from build123d import *

# Parameters (mm, degrees)
F1_DEPTH  = 20
F2_START  = 10
F1_FACE_R = 1.5
F2_DEPTH  = 10


# Not quite as in the source:
# - a feature names something its author has since deleted; it is built from what else it names


with BuildPart() as f1:
    # F0 (on Top) → F1 (new body)
    with BuildSketch(Plane.XY):
        Polygon((8, 0), (0, 0), (0, -2), (10, -2), (10, 4), (10, 10), (0, 10), (0, 8), (8, 8), align=None)
        with BuildLine():
            Line((16, 2.5), (16, -2))
            ThreePointArc((16, -2), (22, 4), (16, 10))
            Line((16, 10), (16, 5.5))
            ThreePointArc((16, 5.5), (17.0606601718, 5.0606601718), (17.5, 4))
            ThreePointArc((17.5, 4), (17.0606601718, 2.9393398282), (16, 2.5))
        make_face()
        with BuildLine():
            ThreePointArc((10, 4), (11.7573593129, -0.2426406871), (16, -2))
            Line((16, -2), (16, 2.5))
            ThreePointArc((16, 2.5), (14.5, 4), (16, 5.5))
            Line((16, 5.5), (16, 10))
            ThreePointArc((16, 10), (11.7573593129, 8.2426406871), (10, 4))
        make_face()
        with BuildLine():
            Line((16, 10), (10, 10))
            Line((10, 10), (10, 4))
            ThreePointArc((10, 4), (11.7573593129, 8.2426406871), (16, 10))
        make_face()
        with BuildLine():
            Line((10, 4), (10, -2))
            Line((10, -2), (16, -2))
            ThreePointArc((16, -2), (11.7573593129, -0.2426406871), (10, 4))
        make_face()
    extrude(amount=F1_DEPTH)

    # F0 (on Top) + F1_face (on face) → F2 (cut)
    with BuildSketch(Plane.XY.offset(F2_START)):
        with BuildLine():
            Line((16, 2.5), (16, -2))
            ThreePointArc((16, -2), (22, 4), (16, 10))
            Line((16, 10), (16, 5.5))
            ThreePointArc((16, 5.5), (17.0606601718, 5.0606601718), (17.5, 4))
            ThreePointArc((17.5, 4), (17.0606601718, 2.9393398282), (16, 2.5))
        make_face()
        with BuildLine():
            ThreePointArc((10, 4), (11.7573593129, -0.2426406871), (16, -2))
            Line((16, -2), (16, 2.5))
            ThreePointArc((16, 2.5), (14.5, 4), (16, 5.5))
            Line((16, 5.5), (16, 10))
            ThreePointArc((16, 10), (11.7573593129, 8.2426406871), (10, 4))
        make_face()
        with BuildLine():
            Line((10, 4), (10, -2))
            Line((10, -2), (16, -2))
            ThreePointArc((16, -2), (11.7573593129, -0.2426406871), (10, 4))
        make_face()
        with BuildLine():
            Line((16, 10), (10, 10))
            Line((10, 10), (10, 4))
            ThreePointArc((10, 4), (11.7573593129, 8.2426406871), (16, 10))
        make_face()
    with BuildSketch(Plane(origin=(12.4841125556, 4, 20), x_dir=(1, 0, 0), z_dir=(0, 0, 1)).offset(F2_START)):
        with BuildLine():
            Line((-4.4841125556, -4), (-12.4841125556, -4))
            Line((-12.4841125556, -4), (-12.4841125556, -6))
            Line((-12.4841125556, -6), (3.5158874444, -6))
            ThreePointArc((3.5158874444, -6), (9.5158874444, 0), (3.5158874444, 6))
            Line((3.5158874444, 6), (-12.4841125556, 6))
            Line((-12.4841125556, 6), (-12.4841125556, 4))
            Line((-12.4841125556, 4), (-4.4841125556, 4))
            Line((-4.4841125556, 4), (-4.4841125556, -4))
        make_face()
        with Locations((3.5158874444, 0)):
            Circle(F1_FACE_R, mode=Mode.SUBTRACT)
    extrude(amount=F2_DEPTH, mode=Mode.SUBTRACT)


solid = f1.part
Source: CAD feature listing. Evaluate the final solid. Frame: model axes, mm. A direction names the side the tool comes from. Give positions to 0.01 mm unless a question says otherwise; leave off trailing zeros. Order: outer loops, then holes, each group sorted by start corner. A loop starts at its lowest first (then second) coordinate and runs counter-clockwise, first axis right, second up. Notation, with made-up numbers: (58, 21) -> (78, 21) arc R18 ccw to (78, 39) -> close; hole circle Ø10 at (41, 35.5). An arc over 180 degrees is marked (long way). Write item = value, one per line.
Q1. Cut plane B-B, the plane x = 17. Output: boundary loops of the cut face in (y, z), and give its area (3 significant figures).
Data:
outline = (-1.92, 0) -> (2.88, 0) -> (2.88, 10) -> (-1.92, 10) -> close; (5.12, 0) -> (9.92, 0) -> (9.92, 10) -> (5.12, 10) -> close
area = 96.0 mm^2
Q2. Set-up query: faces 1 (the face through (8, 4, 10)), 2 (the face through (10, 4, 15)), 3 (the face through (8.3, 5.4, 20)). Return all of +Z, -Z, +X, -X, +Y, -Y with unobstructed straight access to the full face (end or side cutting, diameter ignored); none if empty.
Data:
face_1 = +Z, -Z, -X
face_2 = +Z, +X, +Y, -Y
face_3 = +Z, +X, -X, +Y, -Y
Q3. Cut plane C-C, the plane z = 11. Output: boundary loops of the cut face in (x, y), and give its area (3 significant figures).
Data:
outline = (0, -2) -> (10, -2) -> (10, 10) -> (0, 10) -> (0, 8) -> (8, 8) -> (8, 0) -> (0, 0) -> close
area = 56.0 mm^2
Q4. Cut plane A-A, the plane z = 8.5. Output: boundary loops of the cut face in (x, y), and give its area (3 significant figures).
Data:
outline = (0, -2) -> (16, -2) arc R6 ccw to (16, 10) -> (0, 10) -> (0, 8) -> (8, 8) -> (8, 0) -> (0, 0) -> close; hole circle Ø3 at (16, 4)
area = 177 mm^2
Q5. Pin query (flat end, axial travel): pin 1 (1 mm diameter, centred on y = 8.5, z = 11, fed in from +X); pin 2 (6 mm diameter, centred on x = 13.5, y = 2.5, fed in from +Z); pin 3 (4 mm diameter, centred on y = 4, z = 14.5, fed in from -X). Return the tip coordinate at first contact, or that it passes through.
Data:
pin_1 = 10
pin_2 = 10
pin_3 = 8
Q6. Cut plane D-D, the plane y = -0.75. Output: boundary loops of the cut face in (x, z).
Data:
outline = (0, 0) -> (19.67, 0) -> (19.67, 10) -> (10, 10) -> (10, 20) -> (0, 20) -> close
Q7. Pull-direction query (Y, two-part tool) for faces 4 (the face through (22, 4, 5)), 5 (the face through (4, 8, 10)), 6 (the face through (6, 10, 10)); classes: released by +Y, released by -Y, zero draft, split by the parting line, or undercut.
Data:
face_4 = split by the parting line
face_5 = undercut
face_6 = released by +Y
Q8. Material intervals for line 1 (Y direction, x = 3.5, z = 11.5); line 2 (Z direction, x = 12.25, y = 9.5); line 3 (X direction, y = 7.5, z = 15.75), sorted ascending. Write a range as from..to.
Data:
line_1 = -2..0, 8..10
line_2 = 0..10
line_3 = 8..10
